```python
from build123d import *

# Parameters (mm, degrees)
SKETCH1_W           = 20
SKETCH1_H           = 100
BOSS_EXTRUDE1_DEPTH = 2
CUT_EXTRUDE1_REACH  = 53.029
SKETCH2_R           = 1.5
SKETCH2_R_2         = 3.5
CHAMFER1_SIZE       = 2


with BuildPart() as part:
    # Sketch1 → Boss-Extrude1 (new body)
    with BuildSketch(Plane.XY):
        Rectangle(SKETCH1_W, SKETCH1_H)
    extrude(amount=BOSS_EXTRUDE1_DEPTH)

    # Sketch2 → Cut-Extrude1 (cut, up to next)
    with BuildSketch(Plane.XY.offset(2), mode=Mode.PRIVATE) as cut_extrude1_sk1:
        with Locations((0, 5)):
            Circle(SKETCH2_R)
    cut_extrude1_tool1 = extrude(cut_extrude1_sk1.sketch, amount=-CUT_EXTRUDE1_REACH, mode=Mode.PRIVATE) & part.part
    # Sketch2 → Cut-Extrude1 (cut, up to next)
    with BuildSketch(Plane.XY.offset(2), mode=Mode.PRIVATE) as cut_extrude1_sk2:
        with Locations((0, -30)):
            Circle(SKETCH2_R_2)
    cut_extrude1_tool2 = extrude(cut_extrude1_sk2.sketch, amount=-CUT_EXTRUDE1_REACH, mode=Mode.PRIVATE) & part.part
    # Sketch2 → Cut-Extrude1 (cut, up to next)
    with BuildSketch(Plane.XY.offset(2), mode=Mode.PRIVATE) as cut_extrude1_sk3:
        with BuildLine():
            ThreePointArc((2.454460226, 34.025), (0, 45.5), (-2.454460226, 34.025))
            ThreePointArc((-2.454460226, 34.025), (0, 32), (2.454460226, 34.025))
        make_face()
    cut_extrude1_tool3 = extrude(cut_extrude1_sk3.sketch, amount=-CUT_EXTRUDE1_REACH, mode=Mode.PRIVATE) & part.part
    add(cut_extrude1_tool1.solids().sort_by_distance((0, 5, 2))[0], mode=Mode.SUBTRACT)
    add(cut_extrude1_tool2.solids().sort_by_distance((0, -30, 2))[0], mode=Mode.SUBTRACT)
    add(cut_extrude1_tool3.solids().sort_by_distance((0, 39.186214, 2))[0], mode=Mode.SUBTRACT)

    # Chamfer1
    chamfer1_edges = [part.edges().sort_by_distance(p)[0] for p in [
        (10, -50, 1),
        (-10, -50, 1),
        (-10, 50, 1),
        (10, 50, 1),
    ]]
    chamfer(chamfer1_edges, length=CHAMFER1_SIZE)


solid = part.part
```
Source: CAD feature listing. Evaluate the final solid. Frame: model axes, mm. A direction names the side the tool comes from. Coordinates: 2 decimals unless noted, no trailing zeros. Order: outer loops, then holes, each group sorted by start corner. A loop starts at its lowest first (then second) coordinate and runs counter-clockwise, first axis right, second up. Notation, with made-up numbers: (8, -29.5) - (47, -29.5) arc R16 cw to (47, -17.5) - close; hole circle Ø8 at (14.5, 60.25). An arc over 180 degrees is marked (long way). One line per item, written item: value.
1) Cut plane A-A on x = 0. Output: boundary loops of the cut face in (y, z).
Computed values:
outline: (-50, 0) - (-33.5, 0) - (-33.5, 2) - (-50, 2) - close; (-26.5, 0) - (3.5, 0) - (3.5, 2) - (-26.5, 2) - close; (6.5, 0) - (32, 0) - (32, 2) - (6.5, 2) - close; (45.5, 0) - (50, 0) - (50, 2) - (45.5, 2) - close
2) Mould query, pull axis X, two halves, no side actions, for faces 1 (the face through (0.228, 45.496, 1.014)), 2 (the face through (0, 1, 2)), 3 (the face through (-10, -1, 1)), 4 (the face through (9, -49, 1)). Classes: released by +X, released by -X, zero draft, split by the parting line, or undercut.
Computed values:
face 1: undercut
face 2: zero draft
face 3: released by -X
face 4: released by +X
3) Ray query, line 1 (X direction, y = 39.5, z = 1); line 2 (Y direction, x = -1.75, z = 0.2); line 3 (Y direction, x = 4, z = 1.45). Return the intervals inside material, ascending. Write a range as [from, to].
Computed values:
line 1: x = [-10, -6], [6, 10]
line 2: y = [-50, -33.03], [-26.97, 32.71], [45.24, 50]
line 3: y = [-50, 35.03], [43.97, 50]
4) Contact query for a flat-ended pin moving along its axis: pin 1 (5.5 mm diameter, centred on x = 0, y = -30, fed in from +Z). Output: stop coordinate, or through.
Computed values:
pin 1: passes through
5) Cut plane C-C on z = 1.4. Output: boundary loops of the cut face in (x, y) (3 decimals).
Computed values:
outline: (-10, -48) - (-8, -50) - (8, -50) - (10, -48) - (10, 48) - (8, 50) - (-8, 50) - (-10, 48) - close; hole circle Ø7 at (0, -30); hole (-2.454, 34.025) arc R2.5 ccw to (2.454, 34.025) arc R6 ccw (long way) to start; hole circle Ø3 at (0, 5)
6) Cut plane D-D on y = 39.5. Output: boundary loops of the cut face in (x, z).
Computed values:
outline: (-10, 0) - (-6, 0) - (-6, 2) - (-10, 2) - close; (6, 0) - (10, 0) - (10, 2) - (6, 2) - close
7) Reachability of faces 5 (the face through (0, -50, 1)), 6 (the face through (0, 32, 1)) from +Z, -Z, +X, -X, +Y, -Y: full face, straight path, thin tool, end or side. Return the list, or none.
Computed values:
face 5: +Z, -Z, +X, -X, -Y
face 6: +Z, -Z
8) Cut plane B-B on y = -30. Output: boundary loops of the cut face in (x, z), plus the area to 3 significant figures.
Computed values:
outline: (-10, 0) - (-3.5, 0) - (-3.5, 2) - (-10, 2) - close; (3.5, 0) - (10, 0) - (10, 2) - (3.5, 2) - close
area: 26.0 mm^2
